Drawing for the job (mm, zero at the part's lowest x, y, z). A direction names the side the tool comes from. Round coordinates to 2 decimals unless told otherwise and drop trailing zeros. Loops run counter-clockwise (first coordinate to the right, second up) from the corner with the lowest first, then second, coordinate; pieces in that order, holes last. Notation, with made-up numbers: M 12.5,58 L 65.5,58 A23 ccw 65.5,81 Z; hole C 87.25,33 d2. An arc over 180 degrees is marked long. Put each result on its own line as item: value. Start each with the question number.
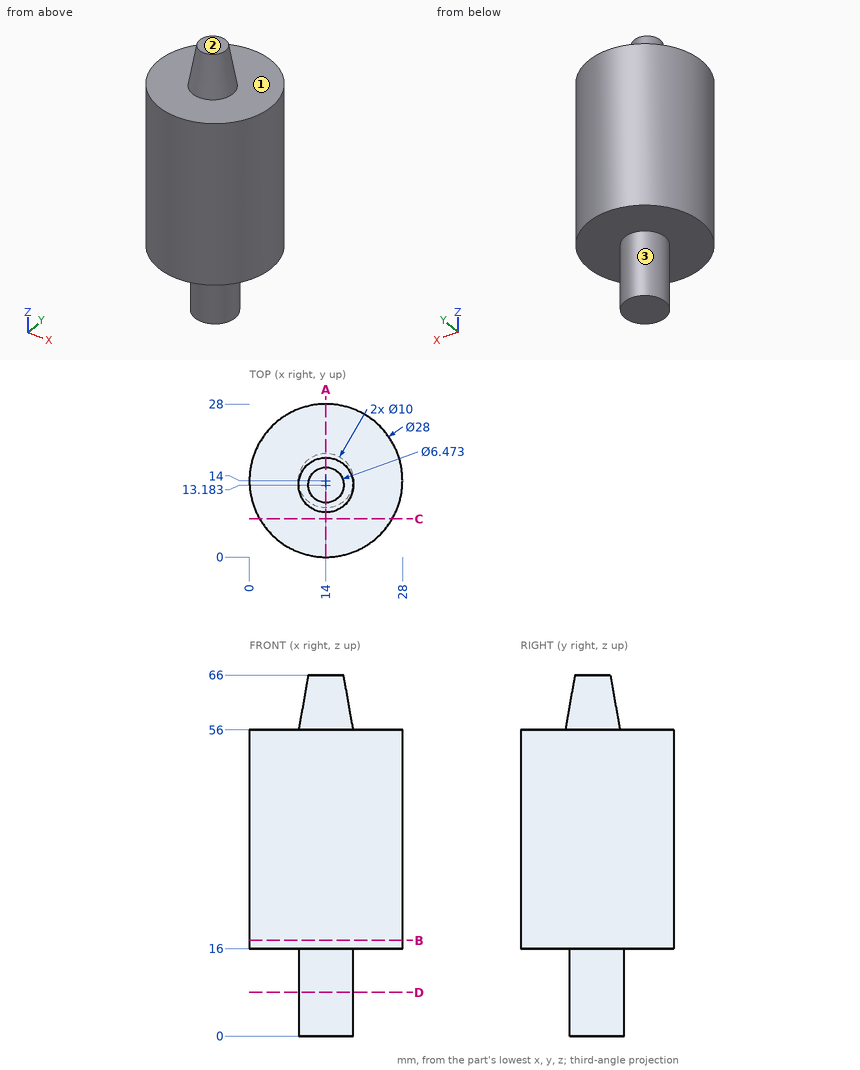
1. Cut at A-A, the plane x = 14. Give the cut face in (y, z).
2. Cut at B-B, the plane z = 17.5. Give the cut face in (x, y), and give its area (3 significant figures).
3. Cut at C-C, the plane y = 7. Give the cut face in (x, z) (1 decimal), and give its area (3 significant figures).
4. Drop flat-ended pins along their axis: pin 1 (6 mm diameter, centred on y = 24.5, z = 50, fed in from +X); pin 2 (6 mm diameter, centred on x = 4.5, y = 23.5, fed in from +Z); pin 3 (1 mm diameter, centred on x = 3, z = 34, fed in from -Y); pin 4 (10 mm diameter, centred on x = 12.5, z = 33.5, fed in from -Y). Give the stop position or say it passes through.
5. Wall check: L1, parallel to Z at x = 13, y = 4; L2, parallel to X at y = 13.75, z = 24.5; L3, parallel to Y at x = 4.5, z = 51 (1 decimal). Give the ranges that are in metal, low to high.
6. Which spindle directions (+Z, -Z, +X, -X, +Y, -Y) get a long thin tool onto all of the face, cutting with end or side? Do the marked faces 1, 2 and 3. Say none if no direction does.
7. Cut at D-D, the plane z = 8. Give the cut face in (x, y).
Results list:
1. outline: M 0,16 L 9,16 L 9,0 L 19,0 L 19,16 L 28,16 L 28,56 L 18.18,56 L 16.42,66 L 9.95,66 L 8.18,56 L 0,56 Z
2. outline: C 14,14 d28
2. area: 616 mm^2
3. outline: M 1.9,16 L 26.1,16 L 26.1,56 L 1.9,56 Z
3. area: 970 mm^2
4. pin 1: stops at x = 25.82
4. pin 2: stops at z = 56
4. pin 3: stops at y = 4.74
4. pin 4: stops at y = 0
5. L1: z = 16 to 56
5. L2: x = 0 to 28
5. L3: y = 3.7 to 24.3
6. face 1: +Z
6. face 2: +Z, +X, -X, +Y, -Y
6. face 3: -Z
7. outline: C 14,14 d10
